Input: part model. Units: mm. Frame: model coordinates. Face numbers are marked on the shaded views. A direction names the side the tool comes from. Round coordinates to 2 decimals unless told otherwise and drop trailing zeros. Loops run counter-clockwise (first coordinate to the right, second up) from the corner with the lowest first, then second, coordinate; pieces in that order, holes last. Notation, with made-up numbers: (-4, -32.5) -> (50, -32.5) arc R26 cw to (50, -3.5) -> close; hole circle Ø6 at (82.5, 40.25). An arc over 180 degrees is marked (long way). Answer in a Markdown table with one row per item. Add a question column.
Q1. Section C-C, the plane z = -9.5. Output: boundary loops of the cut face in (x, y), and give its area (3 significant figures).
Q2. Reachability of the marked faces 1, 2, 3, 4 and 5 from +Z, -Z, +X, -X, +Y, -Y: full face, straight path, thin tool, end or side. Return the list, or none.
Q3. Section B-B, the plane x = -7. Output: boundary loops of the cut face in (y, z), and give its area (3 significant figures).
Q4. Ray query, L1, parallel to X at y = 5, z = 2; L2, parallel to Z at x = -6.5, y = 1.5; L3, parallel to X at y = 2.3, z = -9.5. Return the intervals inside material, ascending. Write a range as from..to.
Q5. Pin query (flat end, axial travel): pin 1 (9.5 mm diameter, centred on x = -18, z = -7, fed in from +Y); pin 2 (1 mm diameter, centred on x = -4, y = 5.5, fed in from -Z); pin 3 (2.5 mm diameter, centred on y = 4.5, z = -2, fed in from -X); pin 4 (2.5 mm diameter, centred on x = 20.5, z = -8, fed in from +Y). Return the tip coordinate at first contact, or that it passes through.
Q6. Mould query, pull axis Z, two halves, no side actions, for the marked faces 6, 7 and 8. Classes: pulls with the +Z half, pulls with the -Z half, needs draft (parallel to the pull), parting line crosses it, or undercut.
Q7. Section A-A, the plane z = 5.5. Output: boundary loops of the cut face in (x, y).
Q8. Section D-D, the plane x = 16. Output: boundary loops of the cut face in (y, z), and give its area (3 significant figures).
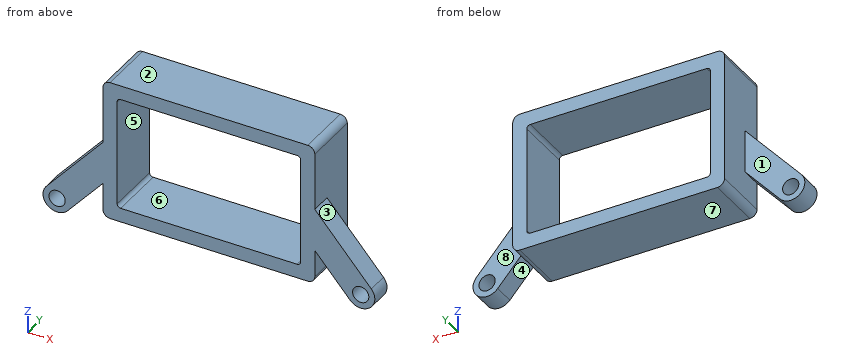
```python
from build123d import *

# Parameters (mm, degrees)
SKETCH1_W           = 30
SKETCH1_H           = 20
SKETCH1_W_2         = 26
SKETCH1_H_2         = 16
SKETCH1_R           = 1.15
BOSS_EXTRUDE1_DEPTH = 3
SKETCH2_W           = 30
SKETCH2_H           = 20
SKETCH2_W_2         = 26
SKETCH2_H_2         = 16
BOSS_EXTRUDE2_DEPTH = 5
FILLET1_R           = 1
FILLET2_R           = 0.5


with BuildPart() as part:
    # Sketch1 → Boss-Extrude1 (new body)
    # profile 1 of 3: a face of its own
    with BuildSketch(Plane(origin=(0, 0, 0), x_dir=(1, 0, 0), z_dir=(0, 1, 0))):
        Rectangle(SKETCH1_W, SKETCH1_H)
        Rectangle(SKETCH1_W_2, SKETCH1_H_2, mode=Mode.SUBTRACT)
    # profile 2 of 3: a face of its own
    with BuildSketch(Plane(origin=(0, 0, 0), x_dir=(1, 0, 0), z_dir=(0, 1, 0))):
        with BuildLine():
            Line((-15, -0.894023008), (-15, 5.15340856))
            Line((-15, 5.15340856), (-20, 10.822875656))
            ThreePointArc((-20, 10.822875656), (-22.822875656, 11), (-23, 8.177124344))
            Line((-23, 8.177124344), (-15, -0.894023008))
        make_face()
        with Locations(Location((-21.5, 9.5, 0), (0, 0, 270))):
            Circle(SKETCH1_R, mode=Mode.SUBTRACT)
    # profile 3 of 3: a face of its own
    with BuildSketch(Plane(origin=(0, 0, 0), x_dir=(1, 0, 0), z_dir=(0, 1, 0))):
        with BuildLine():
            Line((20, 10.822875656), (15, 5.15340856))
            Line((15, 5.15340856), (15, -0.894023008))
            Line((15, -0.894023008), (23, 8.177124344))
            ThreePointArc((23, 8.177124344), (22.822875656, 11), (20, 10.822875656))
        make_face()
        with Locations(Location((21.5, 9.5, 0), (0, 0, 270))):
            Circle(SKETCH1_R, mode=Mode.SUBTRACT)
    extrude(amount=BOSS_EXTRUDE1_DEPTH)

    # Sketch2 → Boss-Extrude2 (add)
    with BuildSketch(Plane(origin=(0, 3, 0), x_dir=(1, 0, 0), z_dir=(0, 1, 0))):
        Rectangle(SKETCH2_W, SKETCH2_H)
        Rectangle(SKETCH2_W_2, SKETCH2_H_2, mode=Mode.SUBTRACT)
    extrude(amount=BOSS_EXTRUDE2_DEPTH)

    # Fillet1
    fillet1_edges = [part.edges().sort_by_distance(p)[0] for p in [
        (-15, 4, 10),
        (-15, 4, -10),
        (15, 4, -10),
        (15, 4, 10),
    ]]
    fillet(fillet1_edges, radius=FILLET1_R)

    # Fillet2
    fillet2_edges = [part.edges().sort_by_distance(p)[0] for p in [
        (13, 4, 8),
        (13, 4, -8),
        (-13, 4, -8),
        (-13, 4, 8),
    ]]
    fillet(fillet2_edges, radius=FILLET2_R)


solid = part.part
```
Answer block:
| question | item | result |
|---|---|---|
| 1 | outline | (-23.5, 0) -> (-22.65, 0) -> (-22.65, 3) -> (-23.5, 3) -> close; (-20.35, 0) -> (-18.83, 0) -> (-18.83, 3) -> (-20.35, 3) -> close; (-14.87, 0) -> (14.87, 0) -> (14.87, 8) -> (-14.87, 8) -> close; (18.83, 0) -> (20.35, 0) -> (20.35, 3) -> (18.83, 3) -> close; (22.65, 0) -> (23.5, 0) -> (23.5, 3) -> (22.65, 3) -> close |
| 1 | area | 252 mm^2 |
| 2 | face 1 | +Z, -Z, -X, +Y |
| 2 | face 2 | +Z, +X, -X, +Y, -Y |
| 2 | face 3 | +Z, +X, +Y, -Y |
| 2 | face 4 | -Z, +Y, -Y |
| 2 | face 5 | +Y, -Y |
| 3 | outline | (0, -10) -> (8, -10) -> (8, -8) -> (0, -8) -> close; (0, 8) -> (8, 8) -> (8, 10) -> (0, 10) -> close |
| 3 | area | 32.0 mm^2 |
| 4 | L1 | -15..-13, 13..15 |
| 4 | L2 | -10..-8, 8..10 |
| 4 | L3 | -23.5..-22.65, -20.35..-18.83, -14.87..14.87, 18.83..20.35, 22.65..23.5 |
| 5 | pin 1 | y = 8 |
| 5 | pin 2 | z = -10 |
| 5 | pin 3 | x = -15 |
| 5 | pin 4 | y = 3 |
| 6 | face 6 | undercut |
| 6 | face 7 | pulls with the -Z half |
| 6 | face 8 | needs draft |
| 7 | outline | (-15, 0) -> (-13, 0) -> (-13, 8) -> (-15, 8) -> close; (13, 0) -> (15, 0) -> (15, 8) -> (13, 8) -> close |
| 8 | outline | (0, -6.29) -> (3, -6.29) -> (3, -0.24) -> (0, -0.24) -> close |
| 8 | area | 18.1 mm^2 |
